```python
from build123d import *

# Parameters (mm, degrees)
F0_R     = 17.5
F0_R_2   = 5
F1_DEPTH = 2
F2_R     = 7.5
F2_R_2   = 5
F3_DEPTH = 10
F4_R     = 1.5
F5_DEPTH = 2


with BuildPart() as f1:
    # F0 (on Top) → F1 (new body)
    with BuildSketch(Plane.XY):
        Circle(F0_R)
        Circle(F0_R_2, mode=Mode.SUBTRACT)
    extrude(amount=-F1_DEPTH)

    # F2 (on face) → F3 (join)
    with BuildSketch(Plane(origin=(0, 0, -2), x_dir=(1, 0, 0), z_dir=(0, 0, -1))):
        Circle(F2_R)
        Circle(F2_R_2, mode=Mode.SUBTRACT)
    extrude(amount=F3_DEPTH)

    # F4 (on face) → F5 (cut, through all)
    with BuildSketch(Plane.XY):
        with Locations((-12.990381, 7.5)):
            Circle(F4_R)
        with Locations((12.990381, 7.5)):
            Circle(F4_R)
        with Locations((0, -15)):
            Circle(F4_R)
    extrude(amount=-F5_DEPTH, mode=Mode.SUBTRACT)


solid = f1.part
```
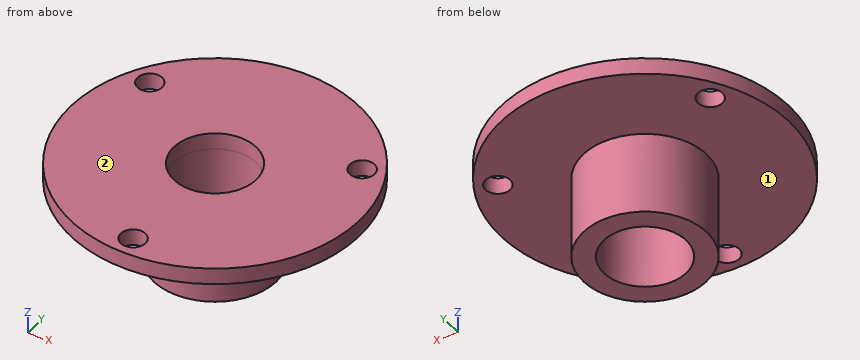
Check sheet for the modelled part. Datum: model origin and axes. Units: mm. Face numbers are marked on the shaded views. A direction names the side the tool comes from. Round coordinates to 2 decimals unless told otherwise and drop trailing zeros. Loops run counter-clockwise (first coordinate to the right, second up) from the corner with the lowest first, then second, coordinate; pieces in that order, holes last. Notation, with made-up numbers: (62, 77) -> (106, 77) arc R22 ccw to (106, 84) -> close; hole circle Ø11 at (-1, -25). An arc over 180 degrees is marked (long way). Answer in a Markdown table with one row per item.
Q1. Sectioned sample at D-D on z = -3.5. Enter the section's corners in (x, y).
Data:
| item | result |
|---|---|
| outline | circle Ø15 at (0, 0); hole circle Ø10 at (0, 0) |
Q2. Sectioned sample at A-A on x = 0. Enter the section's corners in (y, z).
Data:
| item | result |
|---|---|
| outline | (-17.5, -2) -> (-16.5, -2) -> (-16.5, 0) -> (-17.5, 0) -> close; (-13.5, -2) -> (-7.5, -2) -> (-7.5, -12) -> (-5, -12) -> (-5, 0) -> (-13.5, 0) -> close; (5, -12) -> (7.5, -12) -> (7.5, -2) -> (17.5, -2) -> (17.5, 0) -> (5, 0) -> close |
Q3. Sectioned sample at C-C on x = 4.5. Enter the section's corners in (y, z).
Data:
| item | result |
|---|---|
| outline | (-16.91, -2) -> (-6, -2) -> (-6, -12) -> (-2.18, -12) -> (-2.18, 0) -> (-16.91, 0) -> close; (2.18, -12) -> (6, -12) -> (6, -2) -> (16.91, -2) -> (16.91, 0) -> (2.18, 0) -> close |
Q4. Thickness scan on L1, parallel to Y at x = 0, z = -1; L2, parallel to Y at x = 0, z = -7.5; L3, parallel to Z at x = -1, y = 13. Record the ranges inside material, lowest first.
Data:
| item | result |
|---|---|
| L1 | y = -17.5 to -16.5, -13.5 to -5, 5 to 17.5 |
| L2 | y = -7.5 to -5, 5 to 7.5 |
| L3 | z = -2 to 0 |
Q5. Set-up check for the marked faces 1 and 2: record each of +Z, -Z, +X, -X, +Y, -Y from which the full face is reachable in a straight line by a thin tool's end or side.
Data:
| item | result |
|---|---|
| face 1 | -Z |
| face 2 | +Z, +X, -X, +Y, -Y |
Q6. Go/stop test with flat-tipped pins: P1, Ø5, axis at x = -12.99, y = 7.5, coming from the +Z side; P2, Ø1.5, axis at x = 5, y = -11.5, coming from the -Z side; P3, Ø2.5, axis at x = 0, y = -15, coming from the +Z side; P4, Ø1.5, axis at x = -6, z = -1.5, coming from the -Y side. Record where each tip stops, or that it passes through.
Data:
| item | result |
|---|---|
| P1 | stops at z = 0 |
| P2 | stops at z = -2 |
| P3 | passes through |
| P4 | stops at y = -16.69 |
Q7. Sectioned sample at B-B on y = 0. Enter the section's corners in (x, z).
Data:
| item | result |
|---|---|
| outline | (-17.5, -2) -> (-7.5, -2) -> (-7.5, -12) -> (-5, -12) -> (-5, 0) -> (-17.5, 0) -> close; (5, -12) -> (7.5, -12) -> (7.5, -2) -> (17.5, -2) -> (17.5, 0) -> (5, 0) -> close |
